from build123d import *

# Parameters (mm, degrees)
F0_W     = 750
F0_H     = 250
F1_DEPTH = 250
F3_T     = -10
F4_W     = 730
F4_H     = 240
F5_DEPTH = 5
F6_R     = 50
F8_W     = 240
F8_H     = 245
F9_DEPTH = 5


# Not quite as in the source:
# - a feature of the source that left no trace in its solid (it failed there, or was rolled back) is left out


with BuildPart() as f1:
    # F0 (on Front) → F1 (new body)
    with BuildSketch(Plane.XZ):
        with Locations((0, 125)):
            Rectangle(F0_W, F0_H)
    extrude(amount=-F1_DEPTH)

    # F2: F1 across plane


with BuildPart() as f1_1:
    add(f1.part)
    add(f1.part.mirror(Plane.XY))

    # F3
    f3_openings = [f1_1.faces().sort_by_distance(p)[0] for p in [
        (0, 0, 0),
        (0, 125, 250),
        (0, 125, -250),
    ]]
    offset(amount=F3_T, openings=f3_openings)

    # F4 (on Top) → F5 (join, symmetric)
    with BuildSketch(Plane.XY):
        with Locations((0, 120)):
            Rectangle(F4_W, F4_H)
    extrude(amount=F5_DEPTH, both=True)

    # F6
    f6_edges = [f1_1.edges().sort_by_distance(p)[0] for p in [
        (-370, 0, 250),
        (370, 0, 250),
    ]]
    fillet(f6_edges, radius=F6_R)

    # F8 (on Right) → F9 (join, symmetric)
    with BuildSketch(Plane.YZ):
        with Locations((120, -127.5)):
            Rectangle(F8_W, F8_H)
    extrude(amount=F9_DEPTH, both=True)


solid = f1_1.part
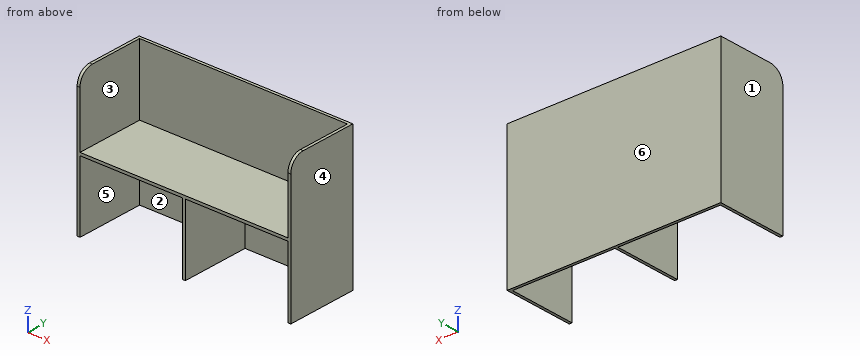
Part model, mm, in its own coordinate system. Face numbers are marked on the shaded views. A direction names the side the tool comes from. Give positions to 0.01 mm unless a question says otherwise; leave off trailing zeros. Order: outer loops, then holes, each group sorted by start corner. A loop starts at its lowest first (then second) coordinate and runs counter-clockwise, first axis right, second up. Notation, with made-up numbers: (35, -11.5) - (93, -11.5) arc R34 ccw to (93, 23.5) - close; hole circle Ø8 at (72.5, -4). An arc over 180 degrees is marked (long way). Use a Markdown table: item, result.
1) Saw through at A-A on z = -215. List the corners of the cut face in (x, y).
Checked values:
| item | result |
|---|---|
| outline | (-375, 0) - (-365, 0) - (-365, 240) - (-5, 240) - (-5, 0) - (5, 0) - (5, 240) - (365, 240) - (365, 0) - (375, 0) - (375, 250) - (-375, 250) - close |
2) 3-axis set-ups, long thin cutter, end or side, ignore diameter. For the marked faces 1, 2 and 3: which of +Z, -Z, +X, -X, +Y, -Y reach the whole face in a straight line?
Checked values:
| item | result |
|---|---|
| face 1 | +Z, -Z, -X, +Y, -Y |
| face 2 | -Z, -Y |
| face 3 | +Z, -Y |
3) Flat gauge pins, fed straight in: P1, Ø2, axis at x = -34, y = 141, coming from the -Z side; P2, Ø3, axis at x = 89.5, y = 43.5, coming from the +Z side; P3, Ø2, axis at x = 13, z = 163.5, coming from the -Y side. Where does each tip first touch, or does it go through?
Checked values:
| item | result |
|---|---|
| P1 | z = -5 |
| P2 | z = 5 |
| P3 | y = 240 |
4) Saw through at C-C on y = 36. List the corners of the cut face in (x, z), plus the area to 3 significant figures.
Checked values:
| item | result |
|---|---|
| outline | (-375, -250) - (-365, -250) - (-365, -5) - (-5, -5) - (-5, -250) - (5, -250) - (5, -5) - (365, -5) - (365, -250) - (375, -250) - (375, 248) - (365, 248) - (365, 5) - (-365, 5) - (-365, 248) - (-375, 248) - close |
| area | 19,700 mm² |
5) Two-plate mould, pull along X, no slides. Class the marked faces 4, 5 and 6: +X half, -X half, draft (parallel to the pull), parting line (faces both ways), or undercut.
Checked values:
| item | result |
|---|---|
| face 4 | +X half |
| face 5 | undercut |
| face 6 | draft |
6) Saw through at D-D on z = 174.5. List the corners of the cut face in (x, y).
Checked values:
| item | result |
|---|---|
| outline | (-375, 0) - (-365, 0) - (-365, 240) - (365, 240) - (365, 0) - (375, 0) - (375, 250) - (-375, 250) - close |
7) Probe L1, parallel to X at y = 129.5, z = 58; L2, parallel to X at y = 122, z = -129; L3, parallel to Y at x = -43, z = 56. List the from-to ranges inside material, lowest first. Write a range as from..to.
Checked values:
| item | result |
|---|---|
| L1 | -375..-365, 365..375 |
| L2 | -375..-365, -5..5, 365..375 |
| L3 | 240..250 |
8) Saw through at B-B on x = -272.5. List the corners of the cut face in (y, z), plus the area to 3 significant figures.
Checked values:
| item | result |
|---|---|
| outline | (0, -5) - (240, -5) - (240, -250) - (250, -250) - (250, 250) - (240, 250) - (240, 5) - (0, 5) - close |
| area | 7,400 mm² |
